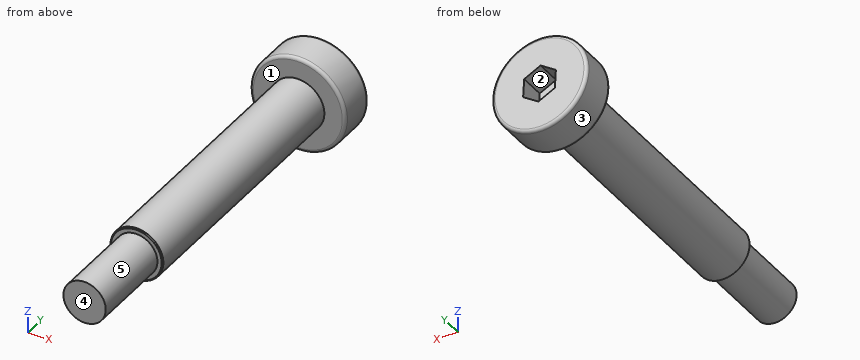
from build123d import *

# Parameters (mm, degrees)
FILLET_2_R          = 0.3
CUT_EXTRUDE_1_DEPTH = 2.4
CHAMFER_2_SIZE      = 0.1


with BuildPart() as part:
    # 草图1 → 旋转1 (revolve)
    with BuildSketch(Plane.XY):
        Polygon((0, 0), (-4.5, 0), (-4.5, -3.5), (-2.5, -3.5), (-2.5, -28.5), (-2, -28.5), (-2, -36.5), (0, -36.5), align=None)
    revolve(axis=Axis((0, -36.5, 0), (0, 1, 0)))

    # 圆角2
    fillet_2_edges = [part.edges().sort_by_distance(p)[0] for p in [
        (4.5, -3.5, 0),
        (4.5, 0, 0),
    ]]
    fillet(fillet_2_edges, radius=FILLET_2_R)

    # 草图2 → 切除-拉伸1 (cut)
    with BuildSketch(Plane(origin=(0, 0, 0), x_dir=(1, 0, 0), z_dir=(0, 1, 0))):
        Polygon((1.448722053, -0.949317867), (1.546494416, 0.779971167), (0.097772363, 1.729289035), (-1.448722053, 0.949317867), (-1.546494416, -0.779971167), (-0.097772363, -1.729289035), align=None)
    extrude(amount=-CUT_EXTRUDE_1_DEPTH, mode=Mode.SUBTRACT)

    # 倒角2
    chamfer_2_edges = [part.edges().sort_by_distance(p)[0] for p in [
        (2.5, -28.5, 0),
    ]]
    chamfer(chamfer_2_edges, length=CHAMFER_2_SIZE)


solid = part.part
Model file for the job. Use its own axes, mm. Face numbers are marked on the shaded views. A direction names the side the tool comes from. Give positions to 0.01 mm unless a question says otherwise; leave off trailing zeros. Loops run counter-clockwise (first coordinate to the right, second up) from the corner with the lowest first, then second, coordinate; pieces in that order, holes last.
1) Tool access for the marked faces 4 and 5: list every direction of +Z, -Z, +X, -X, +Y, -Y with a clear straight run to the whole face (end or side of a thin tool).
2) Pull direction X, two halves, no side cores. Call the marked faces 1, 2 and 3: +X half, -X half, draft (parallel to the pull), parting line (faces both ways), or undercut.
3) Saw through at A-A (z = 0). Write the cut outline in (x, y), plus the area to 3 significant figures.
4) Saw through at B-B (y = -29). Write the cut outline in (x, z), plus the area to 3 significant figures.
5) Wall check: line 1 (Z direction, x = -1.5, y = -17); line 2 (Y direction, x = -2.5, z = 3); line 3 (Y direction, x = -2, z = 1.25). Give the ranges that are in metal, low to high.
6) Saw through at C-C (y = -6.5). Write the cut outline in (x, z), plus the area to 3 significant figures.
7) Flat gauge pins, fed straight in: pin 1 Ø3 at (y, z) = (-21, -1.5) entering from -X; pin 2 Ø4 at (x, y) = (-0.5, -17) entering from +Z; pin 3 Ø3.5 at (x, z) = (0, 0.5) entering from +Y; pin 4 Ø1.5 at (x, y) = (-2.5, -21.5) entering from +Z. Where does each tip first touch, or does it go through?
Answer block:
1. face 4: +Z, -Z, +X, -X, -Y
1. face 5: -Y
2. face 1: draft
2. face 2: undercut
2. face 3: parting line
3. outline: (-4.5, -3.2) arc R0.3 ccw to (-4.2, -3.5) - (-2.5, -3.5) - (-2.5, -28.4) - (-2.4, -28.5) - (-2, -28.5) - (-2, -36.5) - (2, -36.5) - (2, -28.5) - (2.4, -28.5) - (2.5, -28.4) - (2.5, -3.5) - (4.2, -3.5) arc R0.3 ccw to (4.5, -3.2) - (4.5, -0.3) arc R0.3 ccw to (4.2, 0) - (1.5, 0) - (1.5, -2.4) - (-1.5, -2.4) - (-1.5, 0) - (-4.2, 0) arc R0.3 ccw to (-4.5, -0.3) - close
3. area: 181 mm2
4. outline: circle Ø4 at (0, 0)
4. area: 12.6 mm2
5. line 1: z = -2 to 2
5. line 2: y = -3.5 to 0
5. line 3: y = -28.5 to 0
6. outline: circle Ø5 at (0, 0)
6. area: 19.6 mm2
7. pin 1: stops at x = -2.5
7. pin 2: stops at z = 2.5
7. pin 3: stops at y = 0
7. pin 4: stops at z = 1.79
